Check sheet for the modelled part. Datum: model origin and axes. Units: mm. Coordinates: 2 decimals unless noted, no trailing zeros. Order: outer loops, then holes, each group sorted by start corner. A loop starts at its lowest first (then second) coordinate and runs counter-clockwise, first axis right, second up.
from build123d import *

# Parameters (mm, degrees)
F0_W     = 200
F0_H     = 200
F1_DEPTH = 5
F3_D     = 13.5
F5_R     = 8


with BuildPart() as f1:
    # F0 (on Top) → F1 (new body)
    with BuildSketch(Plane.XY):
        with Locations((100, 100)):
            Rectangle(F0_W, F0_H)
    extrude(amount=F1_DEPTH)

    # F3 (through all)
    with Locations(Plane(origin=(0, 0, 0), x_dir=(1, 0, 0), z_dir=(0, 0, -1))):
        with Locations((20, -20), (180, -20), (20, -180), (180, -180)):
            Hole(F3_D / 2)

    # F8: sweep along a path in F7
    with BuildLine(Plane.XZ.offset(-100)) as f8_path:
        Line((118, 5), (118, 25))
        ThreePointArc((118, 25), (100, 43), (82, 25))
        Line((82, 25), (82, 5))
    # F5 (on face) → F8 (sweep)
    with BuildSketch(Plane.XY.offset(5)):
        with Locations((118, 100)):
            Circle(F5_R)
    sweep(path=f8_path.line)


solid = f1.part
(1) Thickness scan on probe 1 along Y at (x, z) = (180, 1.3); probe 2 along Z at (x, y) = (132, 73.5). Record the ranges inside material, lowest first.
Filled in:
probe 1: y = 0 to 13.25, 26.75 to 173.25, 186.75 to 200
probe 2: z = 0 to 5
(2) Cross-section at C-C (y = 100). Enter the section's corners in (x, z).
Filled in:
outline: (0, 0) - (200, 0) - (200, 5) - (126, 5) - (126, 25) arc R26 ccw to (74, 25) - (74, 5) - (0, 5) - close; hole (90, 5) - (110, 5) - (110, 25) arc R10 ccw to (90, 25) - close
(3) Cross-section at A-A (y = 180). Enter the section's corners in (x, z), and give its area (3 significant figures).
Filled in:
outline: (0, 0) - (13.25, 0) - (13.25, 5) - (0, 5) - close; (26.75, 0) - (173.25, 0) - (173.25, 5) - (26.75, 5) - close; (186.75, 0) - (200, 0) - (200, 5) - (186.75, 5) - close
area: 865 mm2
(4) Release check for a two-part mould opening along Z. For faces 1 (the cylindrical face through (88.349, 95.132, 14.86)), 2 (the cylindrical face through (125.39, 96.94, 15.14)), 3 (the cylindrical face through (176.37, 174.31, 2.54)), 4 (the flat face through (99, 101, 0)) record: +Z half, -Z half, draft (parallel to the pull), parting line (faces both ways), or undercut.
Filled in:
face 1: undercut
face 2: undercut
face 3: draft
face 4: -Z half
(5) Cross-section at D-D (x = 62). Enter the section's corners in (y, z), and give its area (3 significant figures).
Filled in:
outline: (0, 0) - (200, 0) - (200, 5) - (0, 5) - close
area: 1,000 mm2
(6) Go/stop test with flat-tipped pins: P1, Ø21.5, axis at x = 180, y = 20, coming from the +Z side; P2, Ø2, axis at x = 104, y = 60.5, coming from the -Z side; P3, Ø11, axis at x = 20, y = 180, coming from the -Z side. Record where each tip stops, or that it passes through.
Filled in:
P1: stops at z = 5
P2: stops at z = 0
P3: passes through
